Geometry check sheet. Reference: the model listing, model coordinates, mm. A direction names the side the tool comes from. Coordinates: 2 decimals unless noted, no trailing zeros. Write each loop counter-clockwise with the first axis right and the second up, starting at its lowest first coordinate (ties: lowest second). Pieces come first, ordered by that corner, then holes.
from build123d import *

# Parameters (mm, degrees)
F0_W     = 38.1
F0_H     = 38.1
F1_DEPTH = 38.1
F4_DEPTH = 38.1
F6_DEPTH = 38.1
F7_W     = 25.4
F7_H     = 7.62
F8_DEPTH = 38.1


with BuildPart() as f1:
    # F0 (on Front) → F1 (new body)
    with BuildSketch(Plane.XZ):
        with Locations((19.05, 19.05)):
            Rectangle(F0_W, F0_H)
    extrude(amount=F1_DEPTH)

    # F3 (on offset) → F4 (cut)
    with BuildSketch(Plane.YZ.offset(38.1)):
        Polygon((-6.35, 38.1), (-31.75, 38.1), (-26.67, 15.875), (-21.59, 28.575), (-16.51, 28.575), (-11.43, 15.875), align=None)
        Polygon((-19.05, 15.875), (-25.4, 0), (-12.7, 0), align=None)
        Polygon((0, 0), (0, 38.1), (-6.35, 0), align=None)
        Polygon((-31.75, 0), (-38.1, 38.1), (-38.1, 0), align=None)
    extrude(amount=-F4_DEPTH, mode=Mode.SUBTRACT)

    # F5 (on Front) → F6 (cut)
    with BuildSketch(Plane.XZ):
        Polygon((38.1, 0), (38.1, 38.1), (31.75, 38.1), align=None)
        Polygon((6.35, 0), (31.75, 0), (26.67, 22.782558), (21.59, 10.082558), (16.51, 10.082558), (11.43, 22.225), align=None)
        Polygon((19.05, 22.225), (25.4, 38.1), (12.7, 38.1), align=None)
        Polygon((0, 38.1), (0, 0), (6.35, 38.1), align=None)
    extrude(amount=F6_DEPTH, mode=Mode.SUBTRACT)

    # F7 (on Top) → F8 (cut)
    with BuildSketch(Plane.XY):
        with Locations((25.4, -11.43)):
            Rectangle(F7_W, F7_H)
        with Locations((12.7, -26.67)):
            Rectangle(F7_W, F7_H)
    extrude(amount=F8_DEPTH, mode=Mode.SUBTRACT)


solid = f1.part
1. Draft check along X on faces 1 (the flat face through (20.302, -18.997, 25.356)), 2 (the flat face through (8.87, -8.926, 26.832)), 3 (the flat face through (3.13, -8.73, 18.78)). Enter one of: released by +X, released by -X, zero draft, split by the parting line, or undercut.
Computed values:
face 1: undercut
face 2: zero draft
face 3: released by -X
2. Sectioned sample at D-D, the plane x = 31. Record the boundary of the cut face in (y, z) (3 decimals), and give its area (3 significant figures).
Computed values:
outline: (-38.1, 38.1) - (-32.311, 3.364) - (-24.055, 3.364) - (-19.05, 15.875) - (-15.24, 6.35) - (-15.24, 25.4) - (-16.51, 28.575) - (-21.59, 28.575) - (-26.67, 15.875) - (-31.75, 38.1) - close; (-7.62, 3.364) - (-5.789, 3.364) - (0, 38.1) - (-6.35, 38.1) - (-7.62, 32.544) - close
area: 594 mm2
3. Sectioned sample at A-A, the plane z = 24.5. Give the number of separate pieces and of enclosed holes in the cut face, and give its area (3 significant figures).
Computed values:
separate pieces: 6
enclosed holes: 0
area: 553 mm2
4. Access from +Z, -Z, +X, -X, +Y, -Y to the whole of each face (thin tool, end or side, straight path). Record for faces 4 (the flat face through (22.2, -33.4, 30.1)), 5 (the flat face through (28.68, -5.61, 13.76)), 6 (the flat face through (25.4, -24, 21)), 7 (the flat face through (8.6, -14, 22.3)), 8 (the flat face through (6, -21, 11)).
Computed values:
face 4: +Z, +Y, -Y
face 5: -Z, +Y, -Y
face 6: +Z, -Z, -X
face 7: +Z, +X, -X
face 8: -Z, +X, -X
5. Gauge pin test, flat ends, axial feed: pin 1 Ø5.5 at (x, z) = (10, 12) entering from -Y; pin 2 Ø2.5 at (y, z) = (-29, 23.5) entering from -X; pin 3 Ø1 at (y, z) = (-31.5, 14.5) entering from -X; pin 4 Ø1 at (y, z) = (-26, 20.5) entering from -X. Record the tip position at first contact, or that the pin passes through.
Computed values:
pin 1: stops at y = -34.21
pin 2: stops at x = 25.4
pin 3: stops at x = 2.33
pin 4: passes through
6. Sectioned sample at C-C, the plane z = 31.5. Record the boundary of the cut face in (x, y).
Computed values:
outline: (5.25, -37) - (15.34, -37) - (15.34, -30.48) - (5.25, -30.48) - close; (5.25, -7.86) - (12.7, -7.86) - (12.7, -7.62) - (15.34, -7.62) - (15.34, -1.1) - (5.25, -1.1) - close; (22.76, -37) - (32.85, -37) - (32.85, -30.24) - (25.4, -30.24) - (25.4, -30.48) - (22.76, -30.48) - close; (22.76, -7.62) - (32.85, -7.62) - (32.85, -1.1) - (22.76, -1.1) - close
7. Sectioned sample at B-B, the plane x = 26. Record the boundary of the cut face in (y, z) (3 decimals), and give its area (3 significant figures).
Computed values:
outline: (-38.1, 38.1) - (-35.268, 21.108) - (-27.866, 21.108) - (-31.75, 38.1) - close; (-24.577, 21.108) - (-15.24, 21.108) - (-15.24, 25.4) - (-16.51, 28.575) - (-21.59, 28.575) - close; (-7.62, 21.108) - (-2.832, 21.108) - (0, 38.1) - (-6.35, 38.1) - (-7.62, 32.544) - close
area: 275 mm2
8. Thickness scan on line 1 along X through (y, z) = (-6.5, 12.5); line 2 along Y through (x, z) = (4.5, 17); line 3 along Y through (x, z) = (25, 20). Record the ranges inside material, lowest first.
Computed values:
line 1: x = 2.08 to 9.21, 15.5 to 22.56, 28.96 to 36.02
line 2: y = -34.58 to -30.48, -22.86 to -11.88, -11.17 to -3.52
line 3: y = -35.08 to -30.48, -22.86 to -15.24, -7.62 to -3.02
